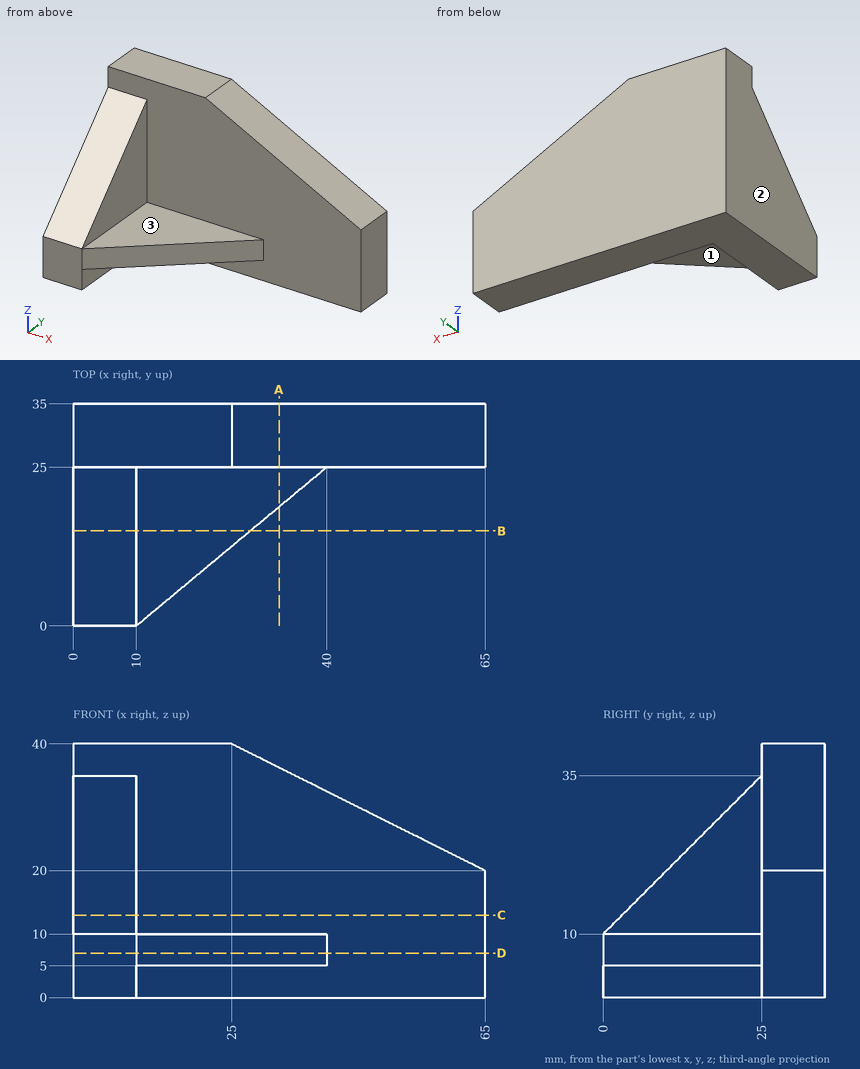
Part print with two shaded views. Sizes in mm from the minimum x, y, z corner. A direction names the side the tool comes from. Round coordinates to 2 decimals unless told otherwise and drop trailing zeros. Write each loop counter-clockwise with the first axis right and the second up, starting at its lowest first coordinate (ties: lowest second). Pieces come first, ordered by that corner, then holes. Notation, with made-up numbers: M -25.5,86.25 L 10.5,86.25 A19 ccw 10.5,104.25 Z; hole C 78.25,-27.5 d4. An arc over 180 degrees is marked long. Answer as CSV lines item,"result". Start each with the question number.
1) Band-saw the part on A-A (x = 32.5). List the corners of the cut face in (y, z), then the cut area to 3 significant figures.
2) Band-saw the part on C-C (z = 13). List the corners of the cut face in (x, y), then the cut area to 3 significant figures.
3) Which spindle directions (+Z, -Z, +X, -X, +Y, -Y) get a long thin tool onto all of the face, cutting with end or side? Do the marked faces 1, 2 and 3. Say none if no direction does.
4) Drill centre lines: L1, parallel to X at y = 20, z = 25.5; L2, parallel to Z at x = 19.5, y = 18.5; L3, parallel to Y at x = 29, z = 36.5. Where is each one in solid material? Low to high.
5) Band-saw the part on D-D (z = 7). List the corners of the cut face in (x, y).
6) Band-saw the part on B-B (y = 15). List the corners of the cut face in (x, z), then the cut area to 3 significant figures.
7) Drop flat-ended pins along their axis: pin 1 (2 mm diameter, centred on x = 9, y = 19.5, fed in from +Z); pin 2 (1.5 mm diameter, centred on y = 11, z = 2.5, fed in from +X); pin 3 (20 mm diameter, centred on x = 32, y = 14.5, fed in from -Z). Give the stop position or say it passes through.
Worked out:
1,outline,"M 18.75,5 L 25,5 L 25,0 L 35,0 L 35,36.25 L 25,36.25 L 25,10 L 18.75,10 Z"
1,area,"394 mm²"
2,outline,"M 0,3 L 10,3 L 10,25 L 65,25 L 65,35 L 0,35 Z"
2,area,"870 mm²"
3,face 1,"-Z, +X, -Y"
3,face 2,"+Z, -Z, -X, +Y, -Y"
3,face 3,"+Z, +X, -Y"
4,L1,"0 to 10"
4,L2,"5 to 10"
4,L3,"25 to 35"
5,outline,"M 0,0 L 10,0 L 40,25 L 65,25 L 65,35 L 0,35 Z"
6,outline,"M 0,0 L 10,0 L 10,5 L 28,5 L 28,10 L 10,10 L 10,25 L 0,25 Z"
6,area,"340 mm²"
7,pin 1,"z = 30.5"
7,pin 2,"x = 10"
7,pin 3,"z = 5"
